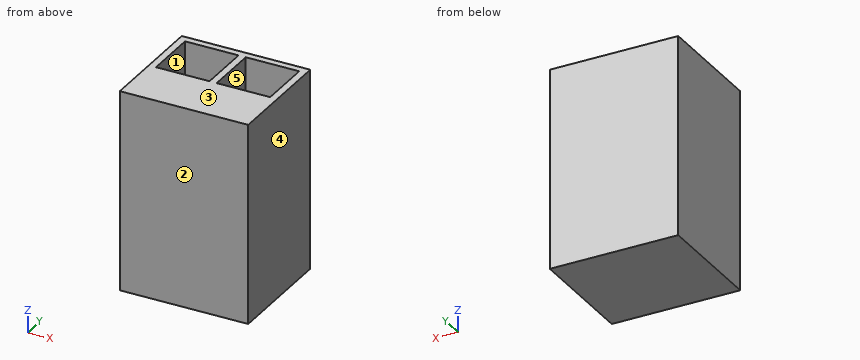
```python
from build123d import *

# Parameters (mm, degrees)
F0_W     = 57.15
F0_H     = 88.9
F1_DEPTH = 50.8
F2_W     = 23.8125
F2_H     = 23.8125
F3_DEPTH = 85.725
F5_W     = 23.8125
F5_H     = 23.8125
F6_DEPTH = 85.725


with BuildPart() as f1:
    # F0 (on Front) → F1 (new body)
    with BuildSketch(Plane.XZ):
        with Locations((-11.298306, 27.606365)):
            Rectangle(F0_W, F0_H)
    extrude(amount=F1_DEPTH)

    # F2 (on face) → F3 (cut)
    with BuildSketch(Plane.XY.offset(72.056365)):
        with Locations((-24.792056, -15.08125)):
            Rectangle(F2_W, F2_H)
    extrude(amount=-F3_DEPTH, mode=Mode.SUBTRACT)

    # F5 (on face) → F6 (cut)
    with BuildSketch(Plane.XY.offset(72.056365)):
        with Locations((2.195444, -15.08125)):
            Rectangle(F5_W, F5_H)
    extrude(amount=-F6_DEPTH, mode=Mode.SUBTRACT)


solid = f1.part
```
Check sheet for the modelled part. Datum: model origin and axes. Units: mm. Face numbers are marked on the shaded views. A direction names the side the tool comes from. Give positions to 0.01 mm unless a question says otherwise; leave off trailing zeros. Loops run counter-clockwise (first coordinate to the right, second up) from the corner with the lowest first, then second, coordinate; pieces in that order, holes last. Notation, with made-up numbers: M 55.5,51 L 71.5,51 A25 ccw 71.5,73 Z; hole C 65.25,86.25 d11. An arc over 180 degrees is marked long. Answer in a Markdown table with one row per item.
1) Cross-section at A-A (z = 4). Enter the section's corners in (x, y) (1 decimal), plus the area to 3 significant figures.
Solutions:
| item | result |
|---|---|
| outline | M -39.9,-50.8 L 17.3,-50.8 L 17.3,0 L -39.9,0 Z; hole M -36.7,-27 L -12.9,-27 L -12.9,-3.2 L -36.7,-3.2 Z; hole M -9.7,-27 L 14.1,-27 L 14.1,-3.2 L -9.7,-3.2 Z |
| area | 1,770 mm^2 |
2) Depth check by flat-ended pin: pin 1 (6 mm diameter, centred on x = 7, z = 34.5, fed in from +Y); pin 2 (12 mm diameter, centred on x = -19, y = -16.5, fed in from +Z). Enter the tip coordinate at first touch or a pass-through.
Solutions:
| item | result |
|---|---|
| pin 1 | stops at y = 0 |
| pin 2 | stops at z = -13.67 |
3) Tool access check on the marked faces 1 and 2. Record the directions out of +Z, -Z, +X, -X, +Y, -Y that give a thin tool (end or side, any length) a straight path to the whole face; none if there is none.
Solutions:
| item | result |
|---|---|
| face 1 | +Z |
| face 2 | +Z, -Z, +X, -X, -Y |
4) Mould release check, pull along X, two halves, no side actions. Record for the marked faces 3, 4 and 5: released by +X, released by -X, zero draft, split by the parting line, or undercut.
Solutions:
| item | result |
|---|---|
| face 3 | zero draft |
| face 4 | released by +X |
| face 5 | undercut |
5) Thickness scan on line 1 (X direction, y = -9.5, z = 15.5); line 2 (Y direction, x = 4, z = -4) (1 decimal); line 3 (Z direction, x = -6, y = -6). Record the ranges inside material, lowest first.
Solutions:
| item | result |
|---|---|
| line 1 | x = -39.87 to -36.7, -12.89 to -9.71, 14.1 to 17.28 |
| line 2 | y = -50.8 to -27, -3.2 to 0 |
| line 3 | z = -16.84 to -13.67 |
6) Cross-section at B-B (x = -1). Enter the section's corners in (y, z) (1 decimal).
Solutions:
| item | result |
|---|---|
| outline | M -50.8,-16.8 L 0,-16.8 L 0,72.1 L -3.2,72.1 L -3.2,-13.7 L -27,-13.7 L -27,72.1 L -50.8,72.1 Z |
7) Cross-section at C-C (y = -20.5). Enter the section's corners in (x, z), plus the area to 3 significant figures.
Solutions:
| item | result |
|---|---|
| outline | M -39.87,-16.84 L 17.28,-16.84 L 17.28,72.06 L 14.1,72.06 L 14.1,-13.67 L -9.71,-13.67 L -9.71,72.06 L -12.89,72.06 L -12.89,-13.67 L -36.7,-13.67 L -36.7,72.06 L -39.87,72.06 Z |
| area | 998 mm^2 |
